from build123d import *

# Parameters (mm, degrees)
CYLINDER095_R           = 2
CYLINDER095_DEPTH       = 10
CYLINDER095_ROLL_ANGLE  = 90
CYLINDER098_R           = 2
CYLINDER098_DEPTH       = 10
CYLINDER098_ROLL_ANGLE  = 90
CYLINDER019_R           = 1.6
CYLINDER019_DEPTH       = 40
CYLINDER019_PITCH_ANGLE = 90
CYLINDER018_R           = 1.6
CYLINDER018_DEPTH       = 40
CYLINDER018_PITCH_ANGLE = 90
CYLINDER017_R           = 1.6
CYLINDER017_DEPTH       = 40
CYLINDER016_R           = 1.6
CYLINDER016_DEPTH       = 70
CYLINDER016_ROLL_ANGLE  = 90
CYLINDER015_R           = 1.6
CYLINDER015_DEPTH       = 40
BOX018_W                = 116
BOX018_H                = 5
BOX018_DEPTH            = 144


with BuildPart() as cylinder372:
    # Cylinder095 → Cylinder095 (new body)
    with BuildSketch(Plane.XY):
        Circle(CYLINDER095_R)
    extrude(amount=CYLINDER095_DEPTH)


with BuildPart() as cylinder372_1:
    # Cylinder095 roll: moved
    add(cylinder372.part.rotate(Axis((0, 0, 0), (1, 0, 0)), CYLINDER095_ROLL_ANGLE))


with BuildPart() as cylinder372_2:
    # Cylinder095 placement: moved
    add(cylinder372_1.part.moved(Location((49, 25, 30))))


with BuildPart() as cylinder375:
    # Cylinder098 → Cylinder098 (new body)
    with BuildSketch(Plane.XY):
        Circle(CYLINDER098_R)
    extrude(amount=CYLINDER098_DEPTH)


with BuildPart() as cylinder375_1:
    # Cylinder098 roll: moved
    add(cylinder375.part.rotate(Axis((0, 0, 0), (1, 0, 0)), CYLINDER098_ROLL_ANGLE))


with BuildPart() as cylinder375_2:
    # Cylinder098 placement: moved
    add(cylinder375_1.part.moved(Location((49, 25, 130))))


with BuildPart() as cylinder100:
    # Cylinder019 → Cylinder019 (new body)
    with BuildSketch(Plane.XY):
        Circle(CYLINDER019_R)
    extrude(amount=CYLINDER019_DEPTH)


with BuildPart() as cylinder100_1:
    # Cylinder019 pitch: moved
    add(cylinder100.part.rotate(Axis((0, 0, 0), (0, 1, 0)), CYLINDER019_PITCH_ANGLE))


with BuildPart() as cylinder100_2:
    # Cylinder019 placement: moved
    add(cylinder100_1.part.moved(Location((-40, 12, 9.5))))


with BuildPart() as fusion011:
    # Cylinder018 → Cylinder018 (new body)
    with BuildSketch(Plane.XY):
        Circle(CYLINDER018_R)
    extrude(amount=CYLINDER018_DEPTH)


with BuildPart() as fusion011_1:
    # Cylinder018 pitch: moved
    add(fusion011.part.rotate(Axis((0, 0, 0), (0, 1, 0)), CYLINDER018_PITCH_ANGLE))


with BuildPart() as fusion011_2:
    # Cylinder018 placement: moved
    add(fusion011_1.part.moved(Location((-40, -7, 2.5))))

    # Fusion011: union Cylinder100
    add(cylinder100_2.part)


with BuildPart() as fusion012:
    # Cylinder017 → Cylinder017 (new body)
    with BuildSketch(Plane(origin=(-27.5, 7, -15), x_dir=(1, 0, 0), z_dir=(0, 0, 1))):
        Circle(CYLINDER017_R)
    extrude(amount=CYLINDER017_DEPTH)

    # Fusion012: union Fusion011
    add(fusion011_2.part)


with BuildPart() as fusion013:
    # Cylinder016 → Cylinder016 (new body)
    with BuildSketch(Plane.XY):
        Circle(CYLINDER016_R)
    extrude(amount=CYLINDER016_DEPTH)


with BuildPart() as fusion013_1:
    # Cylinder016 roll: moved
    add(fusion013.part.rotate(Axis((0, 0, 0), (1, 0, 0)), CYLINDER016_ROLL_ANGLE))


with BuildPart() as fusion013_2:
    # Cylinder016 placement: moved
    add(fusion013_1.part.moved(Location((-24, 39, 6))))

    # Fusion013: union Fusion012
    add(fusion012.part)


with BuildPart() as cylinder008:
    # Cylinder015 → Cylinder015 (new body)
    with BuildSketch(Plane(origin=(-20.5, -12, -15), x_dir=(1, 0, 0), z_dir=(0, 0, 1))):
        Circle(CYLINDER015_R)
    extrude(amount=CYLINDER015_DEPTH)


with BuildPart() as face_corner_holes003:
    # Fusion017 base: copy of Cylinder008
    add(cylinder008.part)

    # Fusion017: union Fusion013
    add(fusion013_2.part)


with BuildPart() as face_corner_holes003_1:
    # Fusion017 placement: moved
    add(face_corner_holes003.part.moved(Location((104, 0, 132))))


with BuildPart() as face_corner_holes012:
    # Fusion026 base: copy of Cylinder008
    add(cylinder008.part)

    # Fusion026: union Fusion013
    add(fusion013_2.part)


with BuildPart() as face_corner_holes012_1:
    # Fusion026 placement: moved
    add(face_corner_holes012.part.moved(Location((0, 0, 132))))


with BuildPart() as face_corner_holes009:
    # Fusion023 base: copy of Cylinder008
    add(cylinder008.part)

    # Fusion023: union Fusion013
    add(fusion013_2.part)


with BuildPart() as face_corner_holes009_1:
    # Fusion023 placement: moved
    add(face_corner_holes009.part.moved(Location((104, 0, 0))))


with BuildPart() as face_corner_holes006:
    # Fusion020 base: copy of Cylinder008
    add(cylinder008.part)

    # Fusion020: union Fusion013
    add(fusion013_2.part)


with BuildPart() as front_a:
    # Box018 → Box018 (new body)
    with BuildSketch(Plane(origin=(-30, 17, 0), x_dir=(1, 0, 0), z_dir=(0, 0, 1))):
        with Locations((58, 2.5)):
            Rectangle(BOX018_W, BOX018_H)
    extrude(amount=BOX018_DEPTH)

    # Cut015: cut face-corner-holes006
    add(face_corner_holes006.part, mode=Mode.SUBTRACT)

    # Cut019: cut face-corner-holes009
    add(face_corner_holes009_1.part, mode=Mode.SUBTRACT)

    # Cut023: cut face-corner-holes012
    add(face_corner_holes012_1.part, mode=Mode.SUBTRACT)

    # Cut026: cut face-corner-holes003
    add(face_corner_holes003_1.part, mode=Mode.SUBTRACT)

    # Cut059: cut Cylinder375
    add(cylinder375_2.part, mode=Mode.SUBTRACT)

    # Cut060: cut Cylinder372
    add(cylinder372_2.part, mode=Mode.SUBTRACT)


solid = front_a.part
Here's how the part is built. I have some questions about the finished solid (model axes, mm). Coordinates: 2 decimals unless noted, no trailing zeros. Order: outer loops, then holes, each group sorted by start corner. A loop starts at its lowest first (then second) coordinate and runs counter-clockwise, first axis right, second up. Notation, with made-up numbers: (29.5, -28) -> (43.5, -28) arc R28 ccw to (43.5, 7) -> close; hole circle Ø7 at (-13.5, 76.5). An arc over 180 degrees is marked (long way). Answer in a Markdown table with one row per item.
(1) I want a section at B-B on x = 80. List the corners of the cut face in (y, z) for me, then the cut area to 3 significant figures.
Answer key:
| item | result |
|---|---|
| outline | (17, 0) -> (22, 0) -> (22, 4.4) -> (17, 4.4) -> close; (17, 7.6) -> (22, 7.6) -> (22, 136.4) -> (17, 136.4) -> close; (17, 139.6) -> (22, 139.6) -> (22, 144) -> (17, 144) -> close |
| area | 688 mm^2 |
(2) I want a section at A-A on z = 130. List the corners of the cut face in (x, y) for me, then the cut area to 3 significant figures.
Answer key:
| item | result |
|---|---|
| outline | (-30, 17) -> (47, 17) -> (47, 22) -> (-30, 22) -> close; (51, 17) -> (86, 17) -> (86, 22) -> (51, 22) -> close |
| area | 560 mm^2 |
(3) Please list where these lines run through material, in increasing order: probe 1 along Z at (x, y) = (80, 20.2); probe 2 along X at (y, z) = (20.9, 138); probe 3 along Z at (x, y) = (49, 20.85).
Answer key:
| item | result |
|---|---|
| probe 1 | 0 to 4.4, 7.6 to 136.4, 139.6 to 144 |
| probe 2 | -30 to -25.6, -22.4 to 78.4, 81.6 to 86 |
| probe 3 | 0 to 28, 32 to 128, 132 to 144 |
(4) Will this pin go through, and if not, where does the flat tip stop? pin 1 Ø2.5 at (x, z) = (80, 138) entering from +Y.
Answer key:
| item | result |
|---|---|
| pin 1 | through |
(5) Thinking about a two-plate mould opening in Z: for faces 1 (the face through (49.923, 19.535, 128.226)), 2 (the face through (27, 20, 144)), 3 (the face through (27, 20, 0)), 4 (the face through (27, 22, 71)), which applies, +Z half, -Z half, draft (parallel to the pull), parting line (faces both ways), or undercut?
Answer key:
| item | result |
|---|---|
| face 1 | undercut |
| face 2 | +Z half |
| face 3 | -Z half |
| face 4 | draft |
